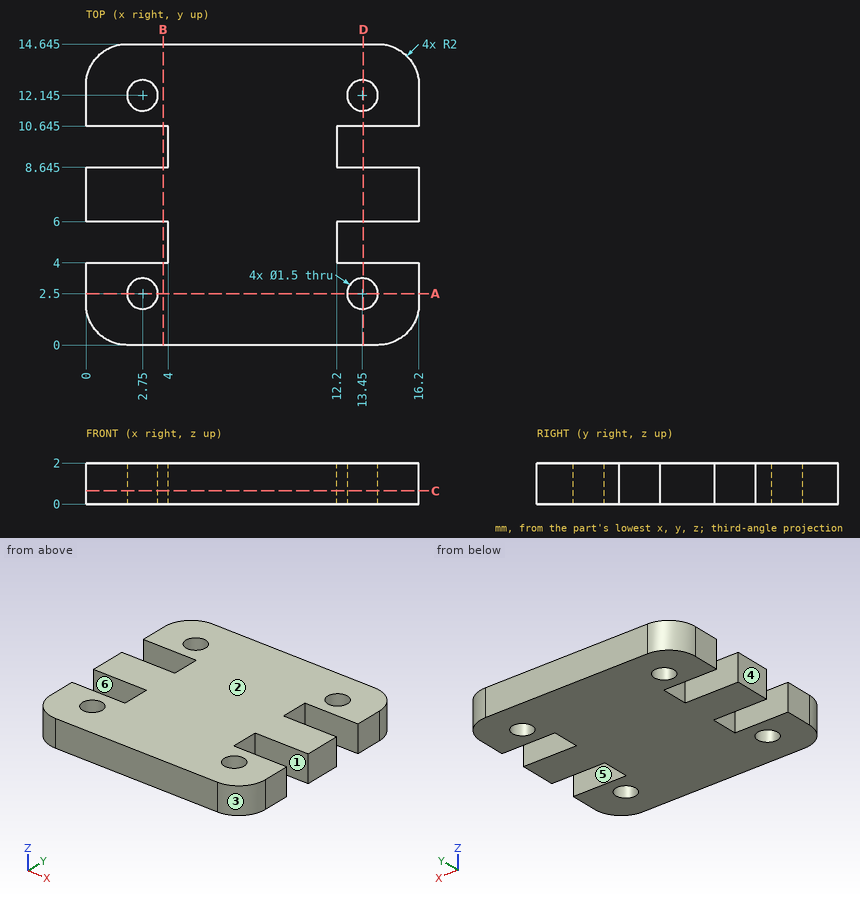
Can you work these out from the drawing? Everything is in mm from the part's minimum corner. A direction names the side the tool comes from. Coordinates: 2 decimals unless noted, no trailing zeros. Loops run counter-clockwise (first coordinate to the right, second up) from the corner with the lowest first, then second, coordinate; pieces in that order, holes last. Notation, with made-up numbers: M 18,-37.5 L 51,-37.5 A22 ccw 51,0.5 Z; hole C 89,1.5 d9. An arc over 180 degrees is marked long. One line per item, written item: value.
1. On a 3-axis mill with a long thin cutter (end or side, diameter ignored), from which of +Z, -Z, +X, -X, +Y, -Y can I reach the whole of each face in a straight line? I mean the marked faces 4, 5 and 6. Say none if no direction works.
Geometry says:
face 4: +Z, -Z, -X, +Y, -Y
face 5: +Z, -Z, +X
face 6: +Z, -Z, -X
2. Thinking about a two-plate mould opening in Y: for the marked faces 1, 2 and 3, which applies, +Y half, -Y half, draft (parallel to the pull), parting line (faces both ways), or undercut?
Geometry says:
face 1: undercut
face 2: draft
face 3: -Y half
3. Imagine slicing it at A-A (y = 2.5). List the corners of the cut face in (x, z) for me.
Geometry says:
outline: M 0,0 L 2,0 L 2,2 L 0,2 Z; M 3.5,0 L 12.7,0 L 12.7,2 L 3.5,2 Z; M 14.2,0 L 16.2,0 L 16.2,2 L 14.2,2 Z
4. Will these pins go through, and if not, where does the flat tip stop? pin 1 Ø1.7 at (x, y) = (13.45, 12.145) entering from +Z; pin 2 Ø0.6 at (y, z) = (9.5, 1) entering from -X; pin 3 Ø0.6 at (y, z) = (9.5, 1) entering from +X; pin 4 Ø0.6 at (x, z) = (1, 1) entering from -Y.
Geometry says:
pin 1: stops at z = 2
pin 2: stops at x = 4
pin 3: stops at x = 12.2
pin 4: stops at y = 0.13
5. Please list where these lines run through material, in increasing order: probe 1 along Y at (x, z) = (2.75, 0.75) (3 decimals); probe 2 along Y at (x, z) = (14.5, 0.2) (3 decimals); probe 3 along X at (y, z) = (12, 0.2).
Geometry says:
probe 1: y = 0 to 1.75, 3.25 to 4, 6 to 8.645, 10.645 to 11.395, 12.895 to 14.645
probe 2: y = 0.023 to 4, 6 to 8.645, 10.645 to 14.622
probe 3: x = 0 to 2.01, 3.49 to 12.71, 14.19 to 16.2
6. Imagine slicing it at D-D (x = 13.5). List the corners of the cut face in (y, z) for me (3 decimals).
Geometry says:
outline: M 0,0 L 1.752,0 L 1.752,2 L 0,2 Z; M 3.248,0 L 4,0 L 4,2 L 3.248,2 Z; M 6,0 L 8.645,0 L 8.645,2 L 6,2 Z; M 10.645,0 L 11.397,0 L 11.397,2 L 10.645,2 Z; M 12.893,0 L 14.645,0 L 14.645,2 L 12.893,2 Z
7. Imagine slicing it at C-C (z = 0.65). List the corners of the cut face in (x, y) for me (3 decimals), and give its area (3 significant figures).
Geometry says:
outline: M 0,2 A2 ccw 2,0 L 14.2,0 A2 ccw 16.2,2 L 16.2,4 L 12.2,4 L 12.2,6 L 16.2,6 L 16.2,8.645 L 12.2,8.645 L 12.2,10.645 L 16.2,10.645 L 16.2,12.645 A2 ccw 14.2,14.645 L 2,14.645 A2 ccw 0,12.645 L 0,10.645 L 4,10.645 L 4,8.645 L 0,8.645 L 0,6 L 4,6 L 4,4 L 0,4 Z; hole C 2.75,2.5 d1.5; hole C 2.75,12.145 d1.5; hole C 13.45,2.5 d1.5; hole C 13.45,12.145 d1.5
area: 195 mm2
8. Imagine slicing it at B-B (x = 3.75). List the corners of the cut face in (y, z) for me (3 decimals), and give its area (3 significant figures).
Geometry says:
outline: M 0,0 L 4,0 L 4,2 L 0,2 Z; M 6,0 L 8.645,0 L 8.645,2 L 6,2 Z; M 10.645,0 L 14.645,0 L 14.645,2 L 10.645,2 Z
area: 21.3 mm2
